Geometry: see drawing. Coordinates: mm, zero at the bounding-box minimum. A direction names the side the tool comes from. Give positions to 0.01 mm unless a question says otherwise; leave off trailing zeros. Write each loop counter-clockwise with the first axis right and the second up, starting at its lowest first coordinate (ties: lowest second). Pieces come first, ordered by that corner, then holes. Notation, with made-up numbers: M 82,-13.5 L 137,-13.5 A20 cw 137,-1.5 Z; hole C 34,-32 d4. An arc over 180 degrees is marked long. Answer as a JSON object with one key per item and string values. Group by question number.
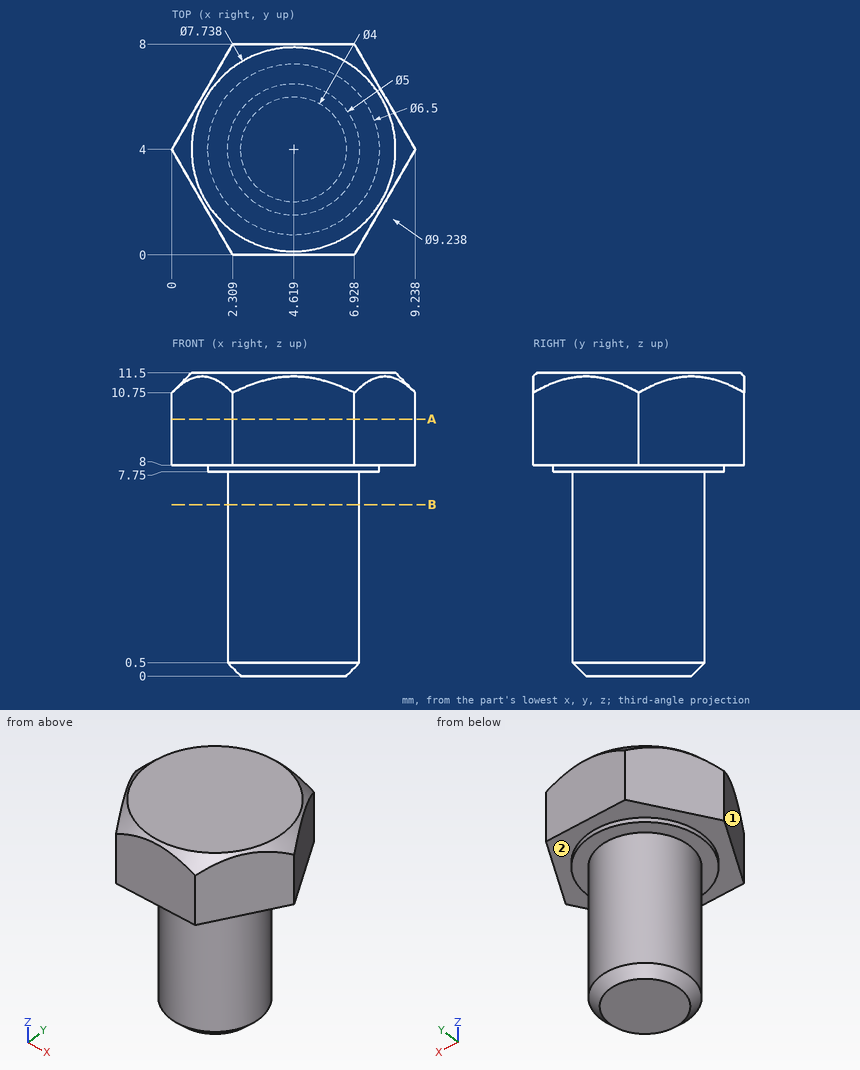
(1) Section A-A, the plane z = 9.75. Return loops of the section in (x, y), plus the area to 3 significant figures.
(2) Access query for the marked faces 1 and 2. Directions: +Z, -Z, +X, -X, +Y, -Y. A direction counts if a zero-diameter tool reaches every point of the face in a straight line with its end or side. Return the directions, or none.
(3) Ray query, L1, parallel to Z at x = 6, y = 6.25; L2, parallel to Y at x = 4.5, z = 1; L3, parallel to Z at x = 5.25, y = 7.25. Return the intervals inside material, ascending. Write a range as [from, to].
(4) Section B-B, the plane z = 6.5. Return loops of the section in (x, y).
(5) Contact query for flat-ended pins moving along their axis: pin 1 Ø3 at (x, z) = (1.5, 4.5) entering from -Y (1 decimal); pin 2 Ø1.5 at (x, z) = (5.5, 2) entering from -Y. Output: stop coordinate, or through.
Reported:
{
 "1": {"outline": "M 0,4 L 2.31,0 L 6.93,0 L 9.24,4 L 6.93,8 L 2.31,8 Z", "area": "55.4 mm2"},
 "2": {"face 1": "+Z, -Z, -X, -Y", "face 2": "-Z"},
 "3": {"L1": "z = [7.75, 11.5]", "L2": "y = [1.5, 6.5]", "L3": "z = [8, 11.5]"},
 "4": {"outline": "C 4.62,4 d5"},
 "5": {"pin 1": "stops at y = 2.1", "pin 2": "stops at y = 1.5"}
}
